The listing builds one solid part. Answer for the finished solid, in the listing's coordinates (mm). Face numbers are marked on the shaded views. A direction names the side the tool comes from. Round coordinates to 2 decimals unless told otherwise and drop trailing zeros. Order: outer loops, then holes, each group sorted by start corner. A loop starts at its lowest first (then second) coordinate and runs counter-clockwise, first axis right, second up. Notation, with made-up numbers: M 7,81.5 L 54,81.5 A33 ccw 54,119.5 Z; hole C 44.5,84.5 d6. An arc over 180 degrees is marked long. Write item = value, one per line. Start each with the question number.
(1) For a pull along X with two mould halves and no side action, classify the marked faces 1, 2 and 3 as released by +X, released by -X, zero draft, split by the parting line, or undercut.
(2) A cutting plane is placed at B-B, the plane z = -4.25. Determine the outline of the cut face in (x, y), and give its area (3 significant figures).
(3) Straight lines are drawn through the part: probe 1 along X at (y, z) = (3, -1); probe 2 along Y at (x, z) = (-3.75, -7); probe 3 along Z at (x, y) = (3.75, -2.5). For each, find the intervals that lie inside material, in ascending order. Write a range as from..to.
(4) A cutting plane is placed at A-A, the plane y = -1. Determine the outline of the cut face in (x, z), and give its area (3 significant figures).
(5) A cutting plane is placed at C-C, the plane x = -0.5. Determine the outline of the cut face in (y, z), and give its area (3 significant figures).
(6) Which of the six approach directions +Z, -Z, +X, -X, +Y, -Y give full straight-line access (tool end or side, diameter ignored) to the marked faces 4, 5 and 6?
(7) Each of these flat-tipped pins is pushed along its axis until it touches: pin 1 (3 mm diameter, centred on x = -1.5, z = -4.5, fed in from -Y); pin 2 (0.8 mm diameter, centred on x = -2.5, y = 2.5, fed in from -Z); pin 3 (1.5 mm diameter, centred on x = -4.5, z = -3, fed in from -Y); pin 4 (1 mm diameter, centred on x = 3.5, z = -7, fed in from +Y). Where does it stop, or does it pass through?
from build123d import *

# Parameters (mm, degrees)
SKETCH_W        = 12.9
SKETCH_H        = 6.5
PAD_DEPTH       = 9.25
FILLET_R        = 0.25
SKETCH001_W     = 9.8
SKETCH001_H     = 0.3
POCKET_DEPTH    = 9.251
SKETCH002_R     = 0.75
POCKET001_DEPTH = 1
PAD001_DEPTH    = 1.95
FILLET001_R     = 0.44


with BuildPart() as part:
    # Sketch → Pad (new body)
    with BuildSketch(Plane.XY):
        Rectangle(SKETCH_W, SKETCH_H)
    extrude(amount=-PAD_DEPTH)

    # Fillet
    fillet_edges = [part.edges().sort_by_distance(p)[0] for p in [
        (6.45, -3.25, -4.625),
        (-6.45, -3.25, -4.625),
        (-6.45, 3.25, -4.625),
        (6.45, 3.25, -4.625),
    ]]
    fillet(fillet_edges, radius=FILLET_R)

    # Sketch001 (on Face2 of Fillet) → Pocket (cut, through all)
    with BuildSketch(Plane.XY):
        with Locations((0, -3.1)):
            Rectangle(SKETCH001_W, SKETCH001_H)
        with Locations((0, 3.1)):
            Rectangle(SKETCH001_W, SKETCH001_H)
    extrude(amount=-POCKET_DEPTH, mode=Mode.SUBTRACT)

    # Sketch002 (on Face4 of Pocket) → Pocket001 (cut)
    with BuildSketch(Plane(origin=(0, 0, -9.25), x_dir=(1, 0, 0), z_dir=(0, 0, -1))):
        with Locations((-2.3, 2.95)):
            Circle(SKETCH002_R)
        with Locations((2.3, 2.95)):
            Circle(SKETCH002_R)
        with Locations((-2.3, -2.95)):
            Circle(SKETCH002_R)
        with Locations((2.3, -2.95)):
            Circle(SKETCH002_R)
    extrude(amount=-POCKET001_DEPTH, mode=Mode.SUBTRACT)

    # Sketch003 → Pad001 (join, symmetric)
    with BuildSketch(Plane.XZ):
        with BuildLine():
            ThreePointArc((-1.85, -9.25), (-2.3, -8.8), (-2.75, -9.25))
            Line((-2.75, -9.25), (-2.75, -9.75))
            ThreePointArc((-2.75, -9.75), (-2.3, -10.2), (-1.85, -9.75))
            Line((-1.85, -9.75), (-1.85, -9.25))
        make_face()
        with BuildLine():
            ThreePointArc((2.75, -9.25), (2.3, -8.8), (1.85, -9.25))
            Line((1.85, -9.25), (1.85, -9.75))
            ThreePointArc((1.85, -9.75), (2.3, -10.2), (2.75, -9.75))
            Line((2.75, -9.75), (2.75, -9.25))
        make_face()
    extrude(amount=PAD001_DEPTH, both=True)

    # Fillet001
    fillet001_edges = [part.edges().sort_by_distance(p)[0] for p in [
        (-2.3, 1.95, -10.2),
        (2.3, 1.95, -10.2),
        (2.3, -1.95, -10.2),
        (-2.3, -1.95, -10.2),
    ]]
    fillet(fillet001_edges, radius=FILLET001_R)


with BuildPart() as part_1:
    # Body placement: moved
    add(part.part.moved(Location((0, 0, -0.3))))


solid = part_1.part
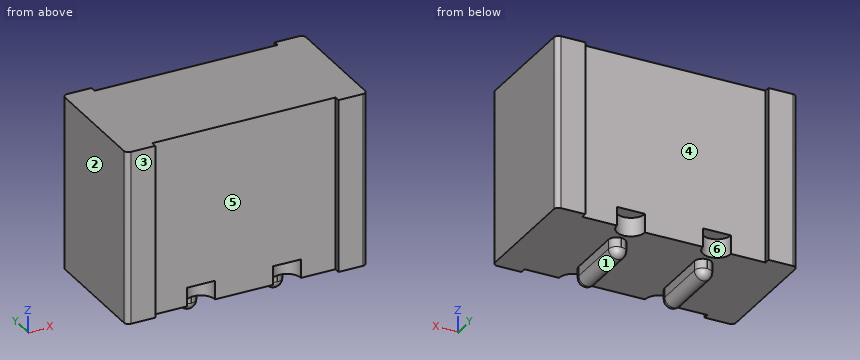
Reported:
q1.face_1 = undercut
q1.face_2 = released by -X
q1.face_3 = zero draft
q2.outline = M -6.45,-3 A0.25 ccw -6.2,-3.25 L -4.9,-3.25 L -4.9,-2.95 L 4.9,-2.95 L 4.9,-3.25 L 6.2,-3.25 A0.25 ccw 6.45,-3 L 6.45,3 A0.25 ccw 6.2,3.25 L 4.9,3.25 L 4.9,2.95 L -4.9,2.95 L -4.9,3.25 L -6.2,3.25 A0.25 ccw -6.45,3 Z
q2.area = 77.9 mm²
q3.probe_1 = -6.45..-4.9, 4.9..6.45
q3.probe_2 = -2.95..2.95
q3.probe_3 = -9.55..-0.3
q4.outline = M -6.45,-9.55 L -2.75,-9.55 L -2.75,-10.05 A0.45 ccw -1.85,-10.05 L -1.85,-9.55 L 1.85,-9.55 L 1.85,-10.05 A0.45 ccw 2.75,-10.05 L 2.75,-9.55 L 6.45,-9.55 L 6.45,-0.3 L -6.45,-0.3 Z
q4.area = 121 mm²
q5.outline = M -2.95,-9.55 L 2.95,-9.55 L 2.95,-0.3 L -2.95,-0.3 Z
q5.area = 54.6 mm²
q6.face_4 = +Z, -Z, +Y
q6.face_5 = +Z, -Z, -Y
q6.face_6 = -Z, +Y
q7.pin_1 = -2.95
q7.pin_2 = -9.55
q7.pin_3 = -3.25
q7.pin_4 = 2.95
